For this review, take the finished solid that the model builds, in its own axes (mm). A direction names the side the tool comes from. Give positions to 0.01 mm unless a question says otherwise; leave off trailing zeros. Order: outer loops, then holes, each group sorted by start corner. A loop starts at its lowest first (then second) coordinate and runs counter-clockwise, first axis right, second up. Notation, with made-up numbers: (13, 9.5) -> (23, 9.5) arc R24 cw to (23, 39.5) -> close; hole circle Ø11 at (84, 89.5). An arc over 180 degrees is marked (long way). Return JSON: item names as keys, results as strings. Group by question number.
1) Insertion check: P1, Ø4, axis at x = -32.5, z = -13.5, coming from the -Y side; P2, Ø1.5, axis at x = -6.5, z = -11, coming from the -Y side; P3, Ø3.5, axis at y = 6, z = -15, coming from the -X side; P4, Ø3, axis at x = -22, y = 14.5, coming from the +Z side. Each pin has a flat end and moves straight along its axis. Give the tip position at first contact, or say it passes through.
2) Add section B-B (z = -9.25). Give the boundary of the cut face in (x, y), then the cut area to 3 significant figures.
3) The part is to be moulded in two halves that separate along X. For faces 1 (the face through (-20.924, 6, -14)), 2 (the face through (-53, 0, -19)), 3 (the face through (-56.124, 4, -8)), say which applies: released by +X, released by -X, zero draft, split by the parting line, or undercut.
4) Add section D-D (x = -27). Give the boundary of the cut face in (y, z), then the cut area to 3 significant figures.
5) Add section C-C (y = 11.25). Give the boundary of the cut face in (x, z), then the cut area to 3 significant figures.
6) For faces 4 (the face through (-50.124, 2, -8)), 5 (the face through (-10.924, 12, -8)), 6 (the face through (-15, 10, -10.176)), list the 3-axis set-ups (+Z, -Z, +X, -X, +Y, -Y) from which the entire face can be reached by the end or side of a thin tool; tool diameter is ignored.
7) Add section A-A (x = -13). Give the boundary of the cut face in (y, z), then the cut area to 3 significant figures.
8) To check wall thickness, follow line 1 along X through (y, z) = (5, -16.5); line 2 along X through (y, z) = (7.5, -19); line 3 along Z through (x, y) = (-49.5, 7.5). State the ranges of each line that lie inside material, in increasing order.
from build123d import *

# Parameters (mm, degrees)
CROQUIS1_W              = 60.2
CROQUIS1_H              = 14
SALIENTE_EXTRUIR1_DEPTH = 20
CROQUIS2_W              = 12
CROQUIS2_H              = 15.4
CORTAR_EXTRUIR1_DEPTH   = 14
CROQUIS3_W              = 10
CROQUIS3_H              = 7
CORTAR_EXTRUIR2_DEPTH   = 20
CORTAR_EXTRUIR3_DEPTH   = 12
CROQUIS5_W              = 12
CROQUIS5_H              = 4
CORTAR_EXTRUIR4_DEPTH   = 3.3


with BuildPart() as part:
    # Croquis1 → Saliente-Extruir1 (new body)
    with BuildSketch(Plane(origin=(0, 0, 0), x_dir=(1, 0, 0), z_dir=(0, 1, 0))):
        with Locations((-26.023666378, 13.176470588)):
            Rectangle(CROQUIS1_W, CROQUIS1_H)
    extrude(amount=SALIENTE_EXTRUIR1_DEPTH)

    # Croquis2 → Cortar-Extruir1 (cut)
    with BuildSketch(Plane.XY.offset(-6.176470588)):
        Polygon((-50.123666378, 0), (-18.623666378, 0), (-18.623666378, 3), (-15.623666378, 3), (-15.623666378, 4.7), (-20.023666378, 4.7), (-51.023666378, 4.7), (-53.123666378, 4.7), (-53.123666378, 3), (-50.123666378, 3), align=None)
        with Locations((-4.923666378, 12.3)):
            Rectangle(CROQUIS2_W, CROQUIS2_H)
    extrude(amount=-CORTAR_EXTRUIR1_DEPTH, mode=Mode.SUBTRACT)

    # Croquis3 → Cortar-Extruir2 (cut)
    with BuildSketch(Plane(origin=(0, 20, 0), x_dir=(1, 0, 0), z_dir=(0, 1, 0))):
        with Locations((-51.123666378, 13.676470588)):
            Rectangle(CROQUIS3_W, CROQUIS3_H)
        with Locations((-15.923666378, 13.676470588)):
            Rectangle(CROQUIS3_W, CROQUIS3_H)
    extrude(amount=-CORTAR_EXTRUIR2_DEPTH, mode=Mode.SUBTRACT)

    # Croquis4 → Cortar-Extruir3 (cut)
    with BuildSketch(Plane(origin=(0, 20, 0), x_dir=(1, 0, 0), z_dir=(0, 1, 0))):
        Polygon((-46.123666378, 17.176470588), (-20.923666378, 17.176470588), (-20.923666378, 10.176470588), (-16.923666378, 10.176470588), (-16.923666378, 6.176470588), (-56.123666378, 6.176470588), (-56.123666378, 10.176470588), (-46.123666378, 10.176470588), align=None)
    extrude(amount=-CORTAR_EXTRUIR3_DEPTH, mode=Mode.SUBTRACT)

    # Croquis5 → Cortar-Extruir4 (cut)
    with BuildSketch(Plane(origin=(0, 8, 0), x_dir=(1, 0, 0), z_dir=(0, 1, 0))):
        with Locations((-33.523666378, 8.176470588)):
            Rectangle(CROQUIS5_W, CROQUIS5_H)
    extrude(amount=-CORTAR_EXTRUIR4_DEPTH, mode=Mode.SUBTRACT)


solid = part.part
Evaluation:
{
 "1": {"P1": "y = 4.7", "P2": "y = 0", "P3": "x = -46.12", "P4": "z = -17.18"},
 "2": {"outline": "(-56.12, 0) -> (-50.12, 0) -> (-50.12, 3) -> (-53.12, 3) -> (-53.12, 4.7) -> (-39.52, 4.7) -> (-39.52, 8) -> (-56.12, 8) -> close; (-27.52, 4.7) -> (-15.62, 4.7) -> (-15.62, 3) -> (-18.62, 3) -> (-18.62, 0) -> (4.08, 0) -> (4.08, 20) -> (1.08, 20) -> (1.08, 4.6) -> (-10.92, 4.6) -> (-10.92, 20) -> (-16.92, 20) -> (-16.92, 8) -> (-27.52, 8) -> close", "area": "351 mm^2"},
 "3": {"face 1": "undercut", "face 2": "zero draft", "face 3": "released by -X"},
 "4": {"outline": "(4.7, -20.18) -> (20, -20.18) -> (20, -17.18) -> (8, -17.18) -> (8, -6.18) -> (4.7, -6.18) -> close", "area": "82.2 mm^2"},
 "5": {"outline": "(-56.12, -20.18) -> (-10.92, -20.18) -> (-10.92, -17.18) -> (-56.12, -17.18) -> close; (-16.92, -10.18) -> (-10.92, -10.18) -> (-10.92, -6.18) -> (-16.92, -6.18) -> close; (1.08, -20.18) -> (4.08, -20.18) -> (4.08, -6.18) -> (1.08, -6.18) -> close", "area": "202 mm^2"},
 "6": {"face 4": "+Z, -Z, -Y", "face 5": "+Z, -Z, +Y", "face 6": "+Y, -Y"},
 "7": {"outline": "(0, -20.18) -> (20, -20.18) -> (20, -17.18) -> (0, -17.18) -> close; (0, -10.18) -> (20, -10.18) -> (20, -6.18) -> (0, -6.18) -> close", "area": "140 mm^2"},
 "8": {"line 1": "-46.12 to -20.92, 1.08 to 4.08", "line 2": "-56.12 to -10.92, 1.08 to 4.08", "line 3": "-20.18 to -17.18, -10.18 to -6.18"}
}
